```python
from build123d import *

# Parameters (mm, degrees)
F0_W      = 54.6
F0_H      = 28.5
F1_DEPTH  = 6.1
F2_R      = 4
F3_R      = 2
F4_W      = 47.8
F4_H      = 22
F5_DEPTH  = 10
F6_W      = 13.2
F6_H      = 22
F7_DEPTH  = 6.1
F8_R      = 1.5
F9_R      = 0.5
F10_DEPTH = 7.5


with BuildPart() as f1:
    # F0 (on Top) → F1 (new body)
    with BuildSketch(Plane.XY):
        with Locations((27.3, 14.25)):
            Rectangle(F0_W, F0_H)
    extrude(amount=F1_DEPTH)

    # F2
    f2_edges = [f1.edges().sort_by_distance(p)[0] for p in [
        (54.6, 0, 3.05),
        (0, 0, 3.05),
        (54.6, 28.5, 3.05),
        (0, 28.5, 3.05),
    ]]
    fillet(f2_edges, radius=F2_R)

    # F3
    f3_edges = [f1.edges().sort_by_distance(p)[0] for p in [
        (54.6, 14.25, 0),
        (53.428427, 1.171573, 0),
        (27.3, 0, 0),
        (53.428427, 27.328427, 0),
        (1.171573, 1.171573, 0),
        (0, 14.25, 0),
        (1.171573, 27.328427, 0),
        (27.3, 28.5, 0),
    ]]
    fillet(f3_edges, radius=F3_R)

    # F4 (on face) → F5 (join)
    with BuildSketch(Plane.XY.offset(6.1)):
        with Locations((27.3, 14.25)):
            Rectangle(F4_W, F4_H)
    extrude(amount=F5_DEPTH)

    # F6 (on face) → F7 (join)
    with BuildSketch(Plane.XY.offset(16.1)):
        with Locations((44.6, 14.25)):
            Rectangle(F6_W, F6_H)
    extrude(amount=F7_DEPTH)

    # F8
    f8_edges = [f1.edges().sort_by_distance(p)[0] for p in [
        (3.4, 3.25, 11.1),
        (20.7, 3.25, 16.1),
        (38, 3.25, 19.15),
        (44.6, 3.25, 22.2),
        (51.2, 3.25, 14.15),
        (51.2, 14.25, 22.2),
        (38, 14.25, 22.2),
        (44.6, 25.25, 22.2),
        (51.2, 25.25, 14.15),
        (20.7, 25.25, 16.1),
        (3.4, 14.25, 16.1),
        (38, 25.25, 19.15),
        (3.4, 25.25, 11.1),
    ]]
    fillet(f8_edges, radius=F8_R)

    # F9 (on face) → F10 (join)
    with BuildSketch(Plane.XY.offset(16.1)):
        with Locations((10.9, 14.25)):
            Circle(F9_R)
        with Locations((14.3549150281, 9.4947174185)):
            Circle(F9_R)
        with Locations((19.9450849719, 11.3110737385)):
            Circle(F9_R)
        with Locations((19.9450849719, 17.1889262615)):
            Circle(F9_R)
        with Locations((14.3549150281, 19.0052825815)):
            Circle(F9_R)
    extrude(amount=F10_DEPTH)


solid = f1.part
```
CAD build for the part. Positions are in the model's coordinates, mm. A direction names the side the tool comes from. Give positions to 0.01 mm unless a question says otherwise; leave off trailing zeros. Order: outer loops, then holes, each group sorted by start corner. A loop starts at its lowest first (then second) coordinate and runs counter-clockwise, first axis right, second up. Notation, with made-up numbers: M 42.25,22 L 98.25,22 A10 ccw 98.25,39 Z; hole C 52,44.5 d11. An arc over 180 degrees is marked long. Put each result on its own line as item: value. Start each with the question number.
(1) Saw through at B-B, the plane x = 6.5. Write the cut outline in (y, z).
(2) Drill centre lines: line 1 along X through (y, z) = (11, 11.25); line 2 along Z through (x, y) = (19, 3); line 3 along Z through (x, y) = (12.5, 19). Where is each one in solid material? Low to high.
(3) Saw through at C-C, the plane y = 22.75. Write the cut outline in (x, z).
(4) Flat gauge pins, fed straight in: pin 1 Ø8.5 at (x, y) = (31, 21) entering from +Z; pin 2 Ø5 at (y, z) = (21, 14.5) entering from -X; pin 3 Ø8 at (x, y) = (45.5, 14) entering from +Z. Where does each tip first touch, or does it go through?
(5) Which spindle directions (+Z, -Z, +X, -X, +Y, -Y) get a long thin tool onto all of the face, cutting with end or side? Do faces 4 (the cylindrical face through (50.77, 24.8, 13.3)), 5 (the flat face through (38, 14, 18)), 6 (the cylindrical face through (22.44, 24.8, 15.67)), 7 (the cylindrical face through (38.43, 3.7, 18.37)). Say none if no direction does.
(6) Saw through at D-D, the plane z = 11.25. Write the cut outline in (x, y).
(7) Mould opens along Y. For faces 1 (the cylindrical face through (44.67, 24.8, 21.77)), 2 (the cylindrical face through (54, 14.39, 0.57)), 3 (the cylindrical face through (19.837, 10.823, 19.798)) say: +Y half, -Y half, draft (parallel to the pull), parting line (faces both ways), or undercut.
(8) Saw through at A-A, the plane z = 21.5. Write the cut outline in (x, y), then the cut area to 3 significant figures.
Check result:
1. outline: M 0,2 A2 ccw 2,0 L 26.5,0 A2 ccw 28.5,2 L 28.5,6.1 L 25.25,6.1 L 25.25,14.6 A1.5 ccw 23.75,16.1 L 4.75,16.1 A1.5 ccw 3.25,14.6 L 3.25,6.1 L 0,6.1 Z
2. line 1: x = 3.4 to 51.2
2. line 2: z = 0 to 6.1
2. line 3: z = 0 to 16.1
3. outline: M 0,2 A2 ccw 2,0 L 52.6,0 A2 ccw 54.6,2 L 54.6,6.1 L 51.2,6.1 L 51.2,20.7 A1.5 ccw 49.7,22.2 L 39.5,22.2 A1.5 ccw 38,20.7 L 38,16.1 L 4.9,16.1 A1.5 ccw 3.4,14.6 L 3.4,6.1 L 0,6.1 Z
4. pin 1: stops at z = 16.1
4. pin 2: stops at x = 3.4
4. pin 3: stops at z = 22.2
5. face 4: +Z, +X, +Y
5. face 5: +Z, +Y, -Y
5. face 6: +Z, -X, +Y
5. face 7: +Z, -X, -Y
6. outline: M 3.4,4.75 A1.5 ccw 4.9,3.25 L 49.7,3.25 A1.5 ccw 51.2,4.75 L 51.2,23.75 A1.5 ccw 49.7,25.25 L 4.9,25.25 A1.5 ccw 3.4,23.75 Z
7. face 1: +Y half
7. face 2: draft
7. face 3: undercut
8. outline: C 10.9,14.25 d1; C 14.35,9.49 d1; C 14.35,19.01 d1; C 19.95,11.31 d1; C 19.95,17.19 d1; M 38.23,4.75 A1.27 ccw 39.5,3.48 L 49.7,3.48 A1.27 ccw 50.97,4.75 L 50.97,23.75 A1.27 ccw 49.7,25.02 L 39.5,25.02 A1.27 ccw 38.23,23.75 Z
8. area: 277 mm2
